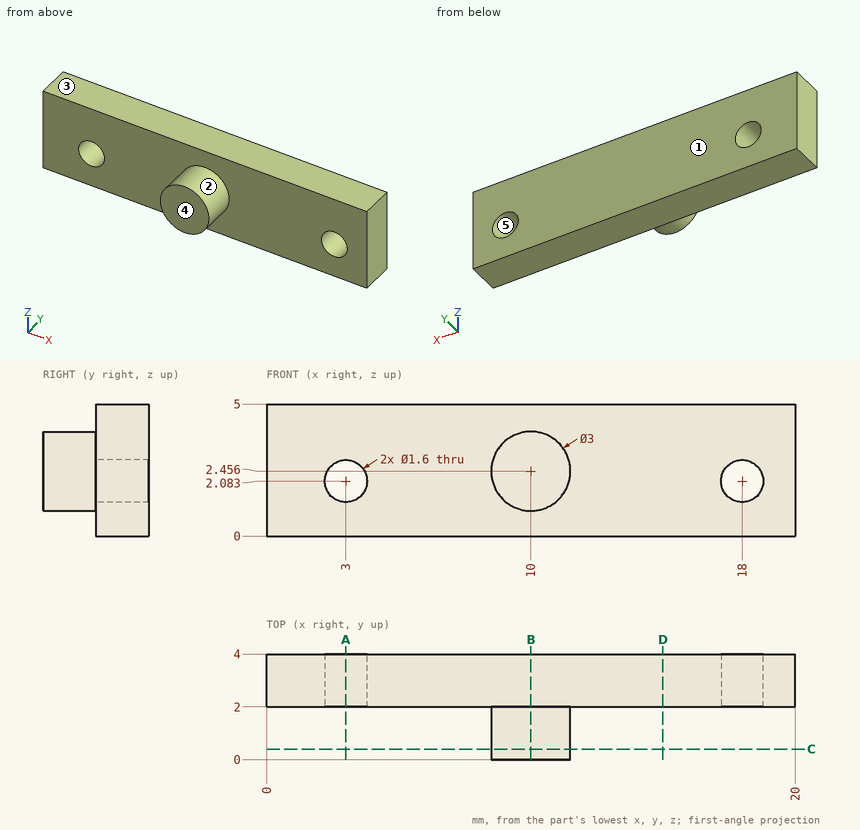
Here's the drawing with two shaded views (mm, measured from the low corner). I have some questions. A direction names the side the tool comes from. Give positions to 0.01 mm unless a question says otherwise; leave off trailing zeros. Write each loop counter-clockwise with the first axis right and the second up, starting at its lowest first coordinate (ties: lowest second). Pieces come first, ordered by that corner, then holes. Notation, with made-up numbers: (-4, -18.75) - (7, -18.75) arc R20 ccw to (7, 7.25) - close; hole circle Ø10 at (-12, -32.75). An arc over 180 degrees is marked (long way). One line per item, written item: value. Start each with the question number.
Item 1: If we mould it in two halves opening along Z, with no side actions, what happens to the marked faces 3, 4 and 5? For each: +Z half, -Z half, draft (parallel to the pull), parting line (faces both ways), or undercut.
Item 2: I'm going to push a flat-ended pin straight in: pin 1 (2 mm diameter, centred on x = 18, z = 2.08, fed in from -Y). Where does the tip first touch, or does it pass through?
Item 3: Imagine slicing it at D-D, the plane x = 15. List the corners of the cut face in (y, z) for me, and give its area (3 significant figures).
Item 4: Imagine slicing it at C-C, the plane y = 0.4. List the corners of the cut face in (x, z) for me.
Item 5: Which directions (+Z, -Z, +X, -X, +Y, -Y) give clear straight access to the entire face, cutting with the end or side of a thin tool? Please do the marked faces 1 and 2.
Item 6: Imagine slicing it at B-B, the plane x = 10. List the corners of the cut face in (y, z) for me, and give its area (3 significant figures).
Item 7: Imagine slicing it at A-A, the plane x = 3. List the corners of the cut face in (y, z) for me.
Item 8: Please list where these lines run through material, in increasing order: line 1 (Z direction, x = 18, y = 3); line 2 (Y direction, x = 6.5, z = 1.8); line 3 (X direction, y = 1.35, z = 1.3) (1 decimal). Write a range as from..to.
Geometry says:
1. face 3: +Z half
1. face 4: draft
1. face 5: undercut
2. pin 1: y = 2
3. outline: (2, 0) - (4, 0) - (4, 5) - (2, 5) - close
3. area: 10.0 mm^2
4. outline: circle Ø3 at (10, 2.46)
5. face 1: +Z, -Z, +X, -X, +Y
5. face 2: -Y
6. outline: (0, 0.96) - (2, 0.96) - (2, 0) - (4, 0) - (4, 5) - (2, 5) - (2, 3.96) - (0, 3.96) - close
6. area: 16.0 mm^2
7. outline: (2, 0) - (4, 0) - (4, 1.28) - (2, 1.28) - close; (2, 2.88) - (4, 2.88) - (4, 5) - (2, 5) - close
8. line 1: 0..1.28, 2.88..5
8. line 2: 2..4
8. line 3: 9..11
